from build123d import *

# Parameters (mm, degrees)
F1_R          = 2.5
F2_DEPTH      = 32.5
F3_R          = 2
F4_DEPTH      = 2.501
F4_DEPTH_BACK = 2.501


with BuildPart() as f2:
    # F1 (on Right) → F2 (new body, symmetric)
    with BuildSketch(Plane.YZ):
        Circle(F1_R)
    extrude(amount=F2_DEPTH, both=True)

    # F3 (on Front) → F4 (cut, two sides)
    with BuildSketch(Plane.XZ) as f4_sk:
        with Locations((-32.5, 0)):
            Circle(F3_R)
        with Locations((32.5, 0)):
            Circle(F3_R)
    extrude(amount=-F4_DEPTH, mode=Mode.SUBTRACT)
    extrude(f4_sk.sketch, amount=F4_DEPTH_BACK, mode=Mode.SUBTRACT)


solid = f2.part
Can you work these out from the model? Positions are in its coordinate system, mm. Give positions to 0.01 mm unless a question says otherwise; leave off trailing zeros. Loops run counter-clockwise (first coordinate to the right, second up) from the corner with the lowest first, then second, coordinate; pieces in that order, holes last. Notation, with made-up numbers: (3.25, 51) -> (60.25, 51) arc R13 cw to (60.25, 69) -> close; hole circle Ø10 at (26.25, 4). An arc over 180 degrees is marked (long way). Return JSON: item names as keys, results as strings.
Q1. I want a section at B-B, the plane x = -27.5. List the corners of the cut face in (y, z) for me.
Checks:
{"outline": "circle Ø5 at (0, 0)"}
Q2. We'd pull the mould along Z, two halves only. Please class faces 1 (the face through (-30.5, 0, 0)), 2 (the face through (0.45, -0.54, -2.44)): released by +Z, released by -Z, zero draft, split by the parting line, or undercut.
Checks:
{"face 1": "undercut", "face 2": "split by the parting line"}
Q3. I need wall thicknesses on probe 1 along Y at (x, z) = (2.5, 0.2); probe 2 along Y at (x, z) = (8.5, -1.5); probe 3 along X at (y, z) = (2.1, 0.15). Which ranges of each line are inside material? Lowest first, please.
Checks:
{"probe 1": "y = -2.49 to 2.49", "probe 2": "y = -2 to 2", "probe 3": "x = -30.51 to 30.51"}
Q4. I want a section at C-C, the plane z = 0. List the corners of the cut face in (x, y) for me.
Checks:
{"outline": "(-30.5, -2.5) -> (30.5, -2.5) -> (30.5, 2.5) -> (-30.5, 2.5) -> close"}
Q5. I want a section at A-A, the plane y = 0. List the corners of the cut face in (x, z) for me.
Checks:
{"outline": "(-32.5, -2.5) -> (32.5, -2.5) -> (32.5, -2) arc R2 cw to (32.5, 2) -> (32.5, 2.5) -> (-32.5, 2.5) -> (-32.5, 2) arc R2 cw to (-32.5, -2) -> close"}
Q6. For pin 1 Ø1.5 at (y, z) = (2, 0) entering from +X; pin 2 Ø1 at (x, z) = (-23, 1.5) entering from +Y, each with a flat end and sliding along its axis, tell me the tip position at first contact or that it passes through.
Checks:
{"pin 1": "stops at x = 30.65", "pin 2": "stops at y = 2.29"}
